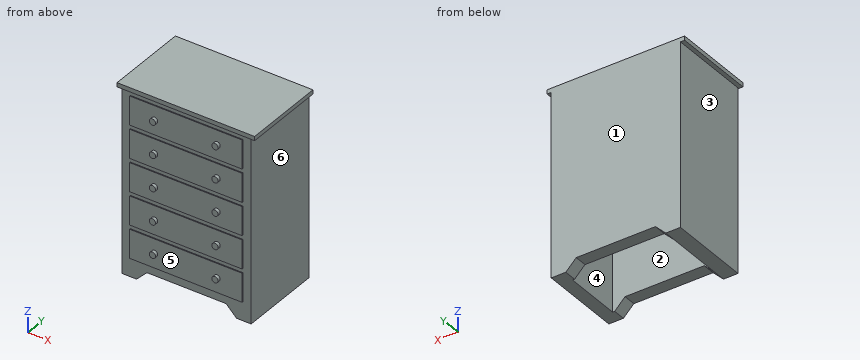
```python
from build123d import *

# Parameters (mm, degrees)
F0_W     = 838.2
F0_H     = 508
F1_DEPTH = 1143
F2_W     = 25.4
F2_H     = 1117.6
F3_DEPTH = 508.001
F2_W_2   = 685.8
F2_H_2   = 175.26
F4_DEPTH = 6.35
F2_R     = 19.05
F5_DEPTH = 19.05
F6_W     = 622.3
F6_H     = 349.25
F7_DEPTH = 1066.8


with BuildPart() as f1:
    # F0 (on Top) → F1 (new body)
    with BuildSketch(Plane.XY):
        Rectangle(F0_W, F0_H)
    extrude(amount=F1_DEPTH)

    # F2 (on face) → F3 (cut, through all)
    with BuildSketch(Plane.XZ.offset(254)):
        with Locations((-406.4, 558.8)):
            Rectangle(F2_W, F2_H)
        with Locations((406.4, 558.8)):
            Rectangle(F2_W, F2_H)
        Polygon((-241.3, 63.5), (-304.8, 0), (304.8, 0), (241.3, 63.5), align=None)
    extrude(amount=-F3_DEPTH, mode=Mode.SUBTRACT)

    # F2 (on face) → F4 (cut)
    with BuildSketch(Plane.XZ.offset(254)):
        Polygon((-393.7, 1117.6), (-393.7, 0), (-304.8, 0), (-241.3, 63.5), (241.3, 63.5), (304.8, 0), (393.7, 0), (393.7, 1117.6), align=None)
        with Locations((0, 201.93)):
            Rectangle(F2_W_2, F2_H_2, mode=Mode.SUBTRACT)
        with Locations((0, 402.59)):
            Rectangle(F2_W_2, F2_H_2, mode=Mode.SUBTRACT)
        with Locations((0, 603.25)):
            Rectangle(F2_W_2, F2_H_2, mode=Mode.SUBTRACT)
        with Locations((0, 803.91)):
            Rectangle(F2_W_2, F2_H_2, mode=Mode.SUBTRACT)
        with Locations((0, 1004.57)):
            Rectangle(F2_W_2, F2_H_2, mode=Mode.SUBTRACT)
    extrude(amount=-F4_DEPTH, mode=Mode.SUBTRACT)

    # F2 (on face) → F5 (join)
    with BuildSketch(Plane.XZ.offset(254)):
        with Locations((-190.5, 1004.57)):
            Circle(F2_R)
        with Locations((190.5, 1004.57)):
            Circle(F2_R)
        with Locations((190.5, 804.0116)):
            Circle(F2_R)
        with Locations((-190.5, 804.0116)):
            Circle(F2_R)
        with Locations((-190.5, 603.4532)):
            Circle(F2_R)
        with Locations((190.5, 603.4532)):
            Circle(F2_R)
        with Locations((190.5, 402.8948)):
            Circle(F2_R)
        with Locations((-190.5, 402.8948)):
            Circle(F2_R)
        with Locations((-190.5, 202.3364)):
            Circle(F2_R)
        with Locations((190.5, 202.3364)):
            Circle(F2_R)
    extrude(amount=F5_DEPTH)

    # F6 (on face) → F7 (cut)
    with BuildSketch(Plane(origin=(0, 0, 0), x_dir=(1, 0, 0), z_dir=(0, 0, -1))):
        with Locations((6.35, -3.175)):
            Rectangle(F6_W, F6_H)
    extrude(amount=-F7_DEPTH, mode=Mode.SUBTRACT)


solid = f1.part
```
Check sheet for the modelled part. Datum: model origin and axes. Units: mm. Face numbers are marked on the shaded views. A direction names the side the tool comes from. Give positions to 0.01 mm unless a question says otherwise; leave off trailing zeros. Order: outer loops, then holes, each group sorted by start corner. A loop starts at its lowest first (then second) coordinate and runs counter-clockwise, first axis right, second up. Notation, with made-up numbers: (-35, 83.5) -> (-11, 83.5) arc R7 ccw to (-11, 93.5) -> close; hole circle Ø1 at (80.25, 14.5). An arc over 180 degrees is marked (long way). Return JSON: item names as keys, results as strings.
1. Set-up check for the marked faces 1, 2 and 3: record each of +Z, -Z, +X, -X, +Y, -Y from which the full face is reachable in a straight line by a thin tool's end or side.
From the geometry:
{"face 1": "+Z, -Z, +X, -X, +Y", "face 2": "-Z", "face 3": "-Z, -X, +Y, -Y"}
2. Mould release check, pull along Y, two halves, no side actions. Record for the marked faces 4, 5 and 6: +Y half, -Y half, draft (parallel to the pull), parting line (faces both ways), or undercut.
From the geometry:
{"face 4": "undercut", "face 5": "-Y half", "face 6": "draft"}
3. Cross-section at B-B, the plane y = 64. Record the cut outline in (x, z), plus the area to 3 significant figures.
From the geometry:
{"outline": "(-419.1, 1117.6) -> (-393.7, 1117.6) -> (-393.7, 0) -> (-304.8, 0) -> (-304.8, 1066.8) -> (317.5, 1066.8) -> (317.5, 0) -> (393.7, 0) -> (393.7, 1117.6) -> (419.1, 1117.6) -> (419.1, 1143) -> (-419.1, 1143) -> close", "area": "237,000 mm^2"}
4. Cross-section at A-A, the plane z = 1004.57. Record the cut outline in (x, y).
From the geometry:
{"outline": "(-393.7, -247.65) -> (-342.9, -247.65) -> (-342.9, -254) -> (-209.55, -254) -> (-209.55, -273.05) -> (-171.45, -273.05) -> (-171.45, -254) -> (171.45, -254) -> (171.45, -273.05) -> (209.55, -273.05) -> (209.55, -254) -> (342.9, -254) -> (342.9, -247.65) -> (393.7, -247.65) -> (393.7, 254) -> (-393.7, 254) -> close; hole (-304.8, -171.45) -> (317.5, -171.45) -> (317.5, 177.8) -> (-304.8, 177.8) -> close"}
5. Cross-section at D-D, the plane z = 864. Record the cut outline in (x, y).
From the geometry:
{"outline": "(-393.7, -247.65) -> (-342.9, -247.65) -> (-342.9, -254) -> (342.9, -254) -> (342.9, -247.65) -> (393.7, -247.65) -> (393.7, 254) -> (-393.7, 254) -> close; hole (-304.8, -171.45) -> (317.5, -171.45) -> (317.5, 177.8) -> (-304.8, 177.8) -> close"}
6. Go/stop test with flat-tipped pins: P1, Ø12, axis at x = 87, z = 671, coming from the -Y side; P2, Ø3, axis at y = -251, z = 1045.5, coming from the +X side; P3, Ø8, axis at y = -108, z = 661.5, coming from the +X side. Record where each tip stops, or that it passes through.
From the geometry:
{"P1": "y = -254", "P2": "x = 342.9", "P3": "x = 393.7"}
7. Material ranges on probe 1 along X at (y, z) = (-105.5, 1059); probe 2 along Y at (x, z) = (-162.5, 1056); probe 3 along X at (y, z) = (-244, 451.5), recorded low to high. Write a range as [from, to].
From the geometry:
{"probe 1": "[-393.7, -304.8], [317.5, 393.7]", "probe 2": "[-254, -171.45], [177.8, 254]", "probe 3": "[-393.7, 393.7]"}
